Geometry check sheet. Reference: the model listing, model coordinates, mm. A direction names the side the tool comes from. Round coordinates to 2 decimals unless told otherwise and drop trailing zeros. Write each loop counter-clockwise with the first axis right and the second up, starting at its lowest first coordinate (ties: lowest second). Pieces come first, ordered by that corner, then holes. Notation, with made-up numbers: (39, 45) -> (67, 45) arc R31 ccw to (67, 72) -> close; hole circle Ø7 at (82.25, -12.5). An arc over 180 degrees is marked (long way). Use a Markdown table: item, result.
```python
from build123d import *

# Parameters (mm, degrees)
BOSS_EXTRUDE1_DEPTH = 5
SKETCH2_R           = 21.5
CUT_EXTRUDE1_DEPTH  = 74.068461049
SKETCH12_R          = 2.9
CUT_EXTRUDE3_DEPTH  = 3
SKETCH13_R          = 1.75
CUT_EXTRUDE4_DEPTH  = 73.958892535


with BuildPart() as part:
    # Sketch1 → Boss-Extrude1 (new body)
    with BuildSketch(Plane.XY):
        with BuildLine():
            Line((25, 65), (-25, 65))
            ThreePointArc((-25, 65), (-30.656854249, 62.656854249), (-33, 57))
            Line((-33, 57), (-33, -57))
            ThreePointArc((-33, -57), (-30.656854249, -62.656854249), (-25, -65))
            Line((-25, -65), (25, -65))
            ThreePointArc((25, -65), (30.656854249, -62.656854249), (33, -57))
            Line((33, -57), (33, 57))
            ThreePointArc((33, 57), (30.656854249, 62.656854249), (25, 65))
        make_face()
    extrude(amount=BOSS_EXTRUDE1_DEPTH)

    # Sketch2 → Cut-Extrude1 (cut, through all)
    with BuildSketch(Plane.XY.offset(5)):
        Circle(SKETCH2_R)
    extrude(amount=-CUT_EXTRUDE1_DEPTH, mode=Mode.SUBTRACT)

    # Sketch12 → Cut-Extrude3 (cut)
    with BuildSketch(Plane.XY.offset(5)):
        with Locations((-27.75, 59.75)):
            Circle(SKETCH12_R)
        with Locations(Location((27.75, 59.75, 0), (0, 0, 180))):
            Circle(SKETCH12_R)
        with Locations(Location((-27.75, -59.75, 0), (0, 0, 180))):
            Circle(SKETCH12_R)
        with Locations((27.75, -59.75)):
            Circle(SKETCH12_R)
    extrude(amount=-CUT_EXTRUDE3_DEPTH, mode=Mode.SUBTRACT)

    # Sketch13 → Cut-Extrude4 (cut, through all)
    with BuildSketch(Plane.XY.offset(2)):
        with Locations((-27.75, 59.75)):
            Circle(SKETCH13_R)
        with Locations(Location((27.75, 59.75, 0), (0, 0, 180))):
            Circle(SKETCH13_R)
        with Locations((27.75, -59.75)):
            Circle(SKETCH13_R)
        with Locations(Location((-27.75, -59.75, 0), (0, 0, 180))):
            Circle(SKETCH13_R)
    extrude(amount=-CUT_EXTRUDE4_DEPTH, mode=Mode.SUBTRACT)


solid = part.part
```
(1) Section check C-C on x = 19. Record the cut outline in (y, z).
A:
| item | result |
|---|---|
| outline | (-65, 0) -> (-10.06, 0) -> (-10.06, 5) -> (-65, 5) -> close; (10.06, 0) -> (65, 0) -> (65, 5) -> (10.06, 5) -> close |
(2) Section check D-D on y = -59.75. Record the cut outline in (x, z), plus the area to 3 significant figures.
A:
| item | result |
|---|---|
| outline | (-32.51, 0) -> (-29.5, 0) -> (-29.5, 2) -> (-30.65, 2) -> (-30.65, 5) -> (-32.51, 5) -> close; (-26, 0) -> (26, 0) -> (26, 2) -> (24.85, 2) -> (24.85, 5) -> (-24.85, 5) -> (-24.85, 2) -> (-26, 2) -> close; (29.5, 0) -> (32.51, 0) -> (32.51, 5) -> (30.65, 5) -> (30.65, 2) -> (29.5, 2) -> close |
| area | 276 mm2 |
(3) Release check for a two-part mould opening along Y. For faces 1 (the face through (-30.719, -62.594, 2.465)), 2 (the face through (-30, -60, 2)), 3 (the face through (33, -1, 2)) record: +Y half, -Y half, draft (parallel to the pull), parting line (faces both ways), or undercut.
A:
| item | result |
|---|---|
| face 1 | -Y half |
| face 2 | undercut |
| face 3 | draft |
(4) Section check B-B on y = 0. Record the cut outline in (x, z).
A:
| item | result |
|---|---|
| outline | (-33, 0) -> (-21.5, 0) -> (-21.5, 5) -> (-33, 5) -> close; (21.5, 0) -> (33, 0) -> (33, 5) -> (21.5, 5) -> close |
(5) Gauge pin test, flat end, axial feed: pin 1 Ø4.5 at (x, y) = (27.75, -59.75) entering from +Z. Record the tip position at first contact, or that the pin passes through.
A:
| item | result |
|---|---|
| pin 1 | stops at z = 2 |
(6) Thickness scan on line 1 (Y direction, x = -26.5, z = 1.9); line 2 (Y direction, x = 27.75, z = 1.5); line 3 (X direction, y = 12, z = 3.3). Record the ranges inside material, lowest first.
A:
| item | result |
|---|---|
| line 1 | y = -64.86 to -60.97, -58.53 to 58.53, 60.97 to 64.86 |
| line 2 | y = -64.51 to -61.5, -58 to 58, 61.5 to 64.51 |
| line 3 | x = -33 to -17.84, 17.84 to 33 |
(7) Section check A-A on z = 3.8. Record the cut outline in (x, y).
A:
| item | result |
|---|---|
| outline | (-33, -57) arc R8 ccw to (-25, -65) -> (25, -65) arc R8 ccw to (33, -57) -> (33, 57) arc R8 ccw to (25, 65) -> (-25, 65) arc R8 ccw to (-33, 57) -> close; hole circle Ø5.8 at (-27.75, -59.75); hole circle Ø5.8 at (-27.75, 59.75); hole circle Ø43 at (0, 0); hole circle Ø5.8 at (27.75, -59.75); hole circle Ø5.8 at (27.75, 59.75) |
(8) Access from +Z, -Z, +X, -X, +Y, -Y to the whole of each face (thin tool, end or side, straight path). Record for faces 4 (the face through (28, -62, 2)), 5 (the face through (26.36, -60.81, 1.01)).
A:
| item | result |
|---|---|
| face 4 | +Z |
| face 5 | +Z, -Z |
